from build123d import *

# Parameters (mm, degrees)
SKETCH_2_W               = 10
SKETCH_2_H               = 12
PATTERN_CIRCULAR_1_COUNT = 5
FILLET_1_R               = 2
CHAMFER_1_SIZE           = 2


with BuildPart() as part:
    # Эскиз1 → Повернуть1 (revolve)
    with BuildSketch(Plane.XY, mode=Mode.PRIVATE) as revolve_1_sk:
        Polygon((35, 0), (75, 0), (75, 12), (40, 12), (40, 50), (25, 50), (25, 25), (35, 25), align=None)
    revolve(revolve_1_sk.sketch.rotate(Axis((0, 0, 0), (0, 1, 0)), 90), axis=Axis((0, 0, 0), (0, 1, 0)))

    # Эскиз2 → Вырез-Повернуть1 (revolve, cut)
    with BuildSketch(Plane.XY, mode=Mode.PRIVATE) as cut_revolve_1_sk:
        with Locations((-60, 6)):
            Rectangle(SKETCH_2_W, SKETCH_2_H)
    cut_revolve_1 = revolve(cut_revolve_1_sk.sketch.rotate(Axis((-55, -2.976144308, 0), (0, 1, 0)), 270), axis=Axis((-55, -2.976144308, 0), (0, 1, 0)), mode=Mode.SUBTRACT)

    # Круговой массив1: Вырез-Повернуть1 ×5 about axis
    pattern_circular_1_axis = Axis((0, 0, 0), (0, 1, 0))
    for i in range(1, PATTERN_CIRCULAR_1_COUNT):
        add(cut_revolve_1.rotate(pattern_circular_1_axis, i * 360 / PATTERN_CIRCULAR_1_COUNT), mode=Mode.SUBTRACT)

    # Скругление1
    fillet_1_edges = [part.edges().sort_by_distance(p)[0] for p in [
        (0, 12, 75),
        (0, 0, 75),
    ]]
    fillet(fillet_1_edges, radius=FILLET_1_R)

    # Фаска1
    chamfer_1_edges = [part.edges().sort_by_distance(p)[0] for p in [
        (0, 50, 40),
    ]]
    chamfer(chamfer_1_edges, length=CHAMFER_1_SIZE)

    # Фаска2: read off the stored shape, not the designer's step
    # Фаска2 outline → Фаска2 (revolve, cut)
    with BuildSketch(Plane.XY):
        Polygon((25, 50), (25, 47), (30.196152423, 50), align=None)
    revolve(axis=Axis((0, 0, 0), (0, 1, 0)), mode=Mode.SUBTRACT)


solid = part.part
For this review, take the finished solid that the model builds, in its own axes (mm). A direction names the side the tool comes from. Round coordinates to 2 decimals unless told otherwise and drop trailing zeros. Write each loop counter-clockwise with the first axis right and the second up, starting at its lowest first coordinate (ties: lowest second). Pieces come first, ordered by that corner, then holes. Notation, with made-up numbers: (-40, -28.75) - (-35, -28.75) arc R16 ccw to (-35, -22.75) - close; hole circle Ø10 at (-3.75, 39). An arc over 180 degrees is marked (long way). Use a Markdown table: item, result.
Q1. The part is to be moulded in two halves that separate along Z. For faces 1 (the flat face through (-28.3, 50, -11.1)), 2 (the cylindrical face through (-1.76, 30.25, 39.96)), 3 (the cylindrical face through (34.168, 12.325, 7.587)), say which applies: pulls with the +Z half, pulls with the -Z half, needs draft (parallel to the pull), parting line crosses it, or undercut.
Derived:
| item | result |
|---|---|
| face 1 | needs draft |
| face 2 | parting line crosses it |
| face 3 | undercut |
Q2. Wall thickness on line 1 along X through (y, z) = (8.5, 0); line 2 along X through (y, z) = (25.5, 1); line 3 along X through (y, z) = (10, 31): over which ranges is each line inside the solid? List them lowest first.
Derived:
| item | result |
|---|---|
| line 1 | x = -75 to -65, -45 to -35, 35 to 75 |
| line 2 | x = -39.99 to -24.98, 24.98 to 39.99 |
| line 3 | x = -68.29 to -16.25, 16.25 to 34.58, 54.41 to 68.29 |
Q3. We need section A-A (x = 0). Give the boundary of the cut face in (y, z), plus the area to 3 significant figures.
Derived:
| item | result |
|---|---|
| outline | (0, -73) arc R2 ccw to (2, -75) - (10, -75) arc R2 ccw to (12, -73) - (12, -40) - (48, -40) - (50, -38) - (50, -30.2) - (47, -25) - (25, -25) - (25, -35) - (0, -35) - close; (0, 35) - (25, 35) - (25, 25) - (47, 25) - (50, 30.2) - (50, 38) - (48, 40) - (12, 40) - (12, 73) arc R2 ccw to (10, 75) - (2, 75) arc R2 ccw to (0, 73) - close |
| area | 1,820 mm2 |
Q4. We need section C-C (y = 21). Give the boundary of the cut face in (x, z), plus the area to 3 significant figures.
Derived:
| item | result |
|---|---|
| outline | circle Ø80 at (0, 0); hole circle Ø70 at (0, 0) |
| area | 1,180 mm2 |
Q5. We need section D-D (y = 41). Give the boundary of the cut face in (x, z), plus the area to 3 significant figures.
Derived:
| item | result |
|---|---|
| outline | circle Ø80 at (0, 0); hole circle Ø50 at (0, 0) |
| area | 3,060 mm2 |
Q6. We need section B-B (z = 0). Give the boundary of the cut face in (x, y), plus the area to 3 significant figures.
Derived:
| item | result |
|---|---|
| outline | (-75, 2) arc R2 ccw to (-73, 0) - (-65, 0) - (-65, 12) - (-73, 12) arc R2 ccw to (-75, 10) - close; (-45, 0) - (-35, 0) - (-35, 25) - (-25, 25) - (-25, 47) - (-30.2, 50) - (-38, 50) - (-40, 48) - (-40, 12) - (-45, 12) - close; (25, 25) - (35, 25) - (35, 0) - (73, 0) arc R2 ccw to (75, 2) - (75, 10) arc R2 ccw to (73, 12) - (40, 12) - (40, 48) - (38, 50) - (30.2, 50) - (25, 47) - close |
| area | 1,580 mm2 |
Q7. Machinability: for faces 4 (the cylindrical face through (54.477, 6.084, -32.935)), 5 (the flat face through (-8, 25, -24)), 6 (the flat face through (31, 12, -31)), which of the approach directions +Z, -Z, +X, -X, +Y, -Y give a long, thin tool a straight path to every point of the face, cutting with its end or side? Answer none if there is none.
Derived:
| item | result |
|---|---|
| face 4 | +Y, -Y |
| face 5 | -Y |
| face 6 | +Y |
Q8. Clearance check with flat-ended pins moving along their axes: pin 1 (16 mm diameter, centred on x = -55, z = 0, fed in from -Y); pin 2 (8 mm diameter, centred on y = 10, z = -28, fed in from -X); pin 3 (10 mm diameter, centred on y = 37.5, z = 34.5, fed in from +X); pin 4 (23 mm diameter, centred on x = 44.5, z = 32.33, fed in from +Y). State where each tip first meets the part, or that it passes through.
Derived:
| item | result |
|---|---|
| pin 1 | passes through |
| pin 2 | stops at x = -71.06 |
| pin 3 | stops at x = 27.01 |
| pin 4 | stops at y = 12 |
